Can you work these out from the drawing? Everything is in mm from the part's minimum corner. A direction names the side the tool comes from. Coordinates: 2 decimals unless noted, no trailing zeros. Order: outer loops, then holes, each group sorted by start corner. A loop starts at its lowest first (then second) coordinate and runs counter-clockwise, first axis right, second up. Notation, with made-up numbers: (-27.75, -17) - (19.25, -17) arc R13 cw to (19.25, 4) - close; hole circle Ø10 at (-5.75, -12.5). An arc over 180 degrees is marked (long way). One line per item, written item: value.
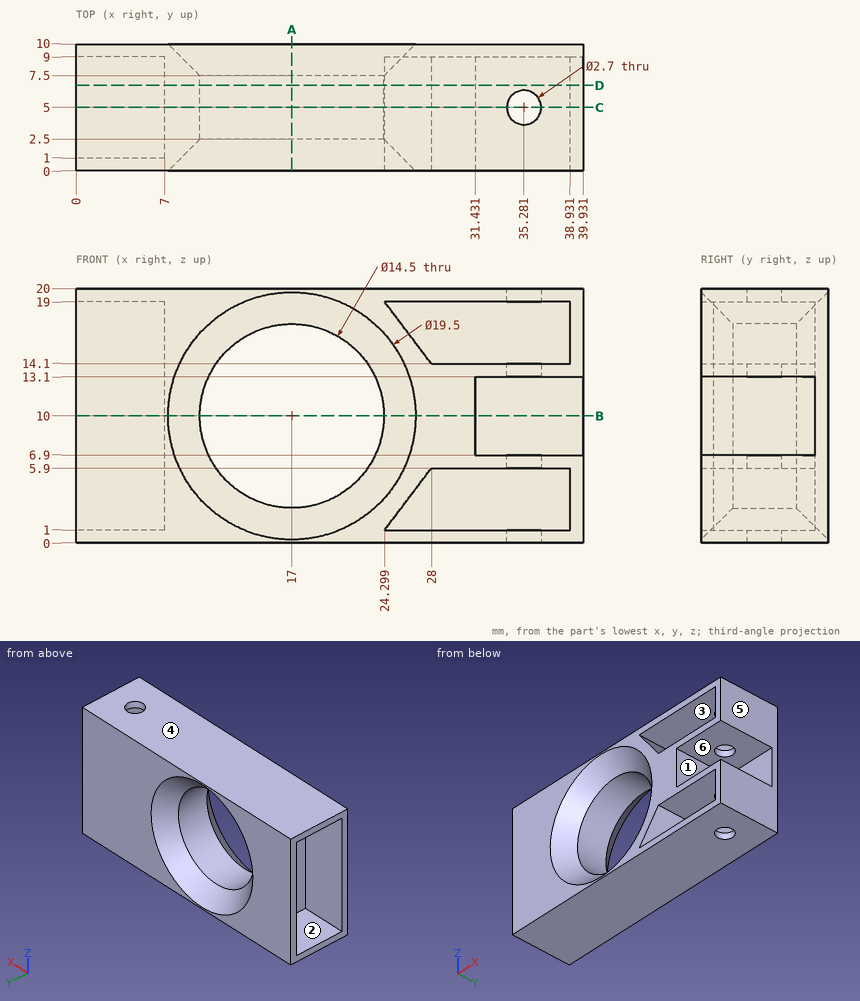
Item 1: Thinking about a two-plate mould opening in Z: for the marked faces 4, 5 and 6, which applies, pulls with the +Z half, pulls with the -Z half, needs draft (parallel to the pull), parting line crosses it, or undercut?
Conclusion:
face 4: pulls with the +Z half
face 5: needs draft
face 6: undercut
Item 2: I want a section at D-D on y = 6.75. Please give me the cut outline in (x, z).
Conclusion:
outline: (0, 0) - (39.93, 0) - (39.93, 6.9) - (31.43, 6.9) - (31.43, 13.1) - (39.93, 13.1) - (39.93, 20) - (0, 20) - (0, 19) - (7, 19) - (7, 1) - (0, 1) - close; hole circle Ø14.5 at (17, 10); hole (24.3, 1) - (38.93, 1) - (38.93, 5.9) - (28, 5.9) - close; hole (24.3, 19) - (28, 14.1) - (38.93, 14.1) - (38.93, 19) - close
Item 3: I want a section at C-C on y = 5. Give the number of separate pieces and of enclosed holes in the cut face, then the cut area to 3 significant figures.
Conclusion:
separate pieces: 3
enclosed holes: 1
area: 319 mm²
Item 4: I want a section at B-B on z = 10. Please give me the cut outline in (x, y), then the cut area to 3 significant figures.
Conclusion:
outline: (0, 0) - (7.25, 0) - (9.75, 2.5) - (9.75, 7.5) - (7.25, 10) - (0, 10) - (0, 9) - (7, 9) - (7, 1) - (0, 1) - close; (24.25, 2.5) - (26.75, 0) - (31.43, 0) - (31.43, 9) - (39.93, 9) - (39.93, 10) - (26.75, 10) - (24.25, 7.5) - close
area: 109 mm²
Item 5: For the marked faces 1, 2 and 3, which set-ups out of +Z, -Z, +X, -X, +Y, -Y let a thin tool reach every point of the face, with its end or its side?
Conclusion:
face 1: +X, -Y
face 2: -X
face 3: -Y
Item 6: I'm going to push flat-ended pins straight in: pin 1 Ø3 at (x, y) = (35.28, 5) entering from -Z; pin 2 Ø3 at (y, z) = (3, 9) entering from +X; pin 3 Ø2.5 at (y, z) = (2.5, 16.5) entering from -X; pin 4 Ø1.5 at (x, z) = (33.5, 16.5) entering from -Y. Where does each tip first touch, or does it pass through?
Conclusion:
pin 1: z = 0
pin 2: x = 31.43
pin 3: x = 7
pin 4: y = 9
Item 7: I want a section at A-A on x = 17. Please give me the cut outline in (y, z), then the cut area to 3 significant figures.
Conclusion:
outline: (0, 0) - (10, 0) - (10, 0.25) - (7.5, 2.75) - (2.5, 2.75) - (0, 0.25) - close; (0, 19.75) - (2.5, 17.25) - (7.5, 17.25) - (10, 19.75) - (10, 20) - (0, 20) - close
area: 42.5 mm²
Item 8: If I drill on probe 1 along Z at (x, y) = (37, 0.75); probe 2 along Y at (x, z) = (5, 17.5); probe 3 along X at (y, z) = (3.65, 10), over which ranges is the centre line in solid material (lowest first)?
Conclusion:
probe 1: 0 to 1, 5.9 to 6.9, 13.1 to 14.1, 19 to 20
probe 2: 0 to 1, 9 to 10
probe 3: 7 to 9.75, 24.25 to 31.43
